Source: CAD feature listing. Evaluate the final solid. Frame: model axes, mm. A direction names the side the tool comes from. Round coordinates to 2 decimals unless told otherwise and drop trailing zeros. Write each loop counter-clockwise with the first axis right and the second up, starting at its lowest first coordinate (ties: lowest second). Pieces come first, ordered by that corner, then holes. Notation, with made-up numbers: M -21.5,32.5 L 1.5,32.5 A11 ccw 1.5,39.5 Z; hole C 9,31 d5. An arc over 180 degrees is marked long. Put each result on its own line as item: value. Start each with the question number.
Autodesk Inventor part; units mm, degrees
ref_plane "YZ Plane" through (0, 0, 0) normal (1, 0, 0) x (0, 1, 0)
ref_plane "XZ Plane" through (0, 0, 0) normal (0, 1, 0) x (-1, 0, 0)
ref_plane "XY Plane" through (0, 0, 0) normal (0, 0, 1) x (1, 0, 0)
sketch "Sketch1" plane through (0, 0, 0) normal (0, 1, 0) x (-1, 0, 0)
  circle A0 centre (0, 0) radius 11.1125
  line L0 (0, -228.6) -> (0, 0) construction
  line L1 (15.875, -228.6) -> (0, -228.6) construction
  circle A1 centre (15.875, -228.6) radius 12.7
  line L2 (25.4, -47.8506) -> (25.4, -198.0228)
  line L3 (57.15, -47.8506) -> (57.15, -181.2924)
  arc A2 (11.2253, 11.2253) -> (-11.2253, -11.2253) centre (0, 0) ccw
  line L4 (-11.2253, -11.2253) -> (25.4, -47.8506)
  arc A3 (57.15, -47.8506) -> (47.8506, -25.4) centre (25.4, -47.8506) ccw
  line L5 (47.8506, -25.4) -> (11.2253, 11.2253)
  circle A4 centre (64.5922, -200.2282) radius 2.8067
  circle A5 centre (64.5922, -256.9718) radius 2.8067
  line L6 (64.5922, -256.9718) -> (64.5922, -200.2282) construction
  line L7 (15.875, -228.6) -> (64.5922, -228.6) construction
  line L8 (15.875, -228.6) -> (-32.8422, -228.6) construction
  circle A6 centre (-32.8422, -228.6) radius 2.8067
  arc A7 (-34.6377, -219.2458) -> (-34.6377, -237.9542) centre (-32.8422, -228.6) ccw
  arc A8 (59.4685, -265.0013) -> (72.1876, -251.2241) centre (64.5922, -256.9718) ccw
  arc A9 (72.1876, -205.9759) -> (65.6336, -190.7603) centre (64.5922, -200.2282) ccw
  line L9 (15.875, -247.65) -> (-34.6377, -237.9542)
  line L10 (15.875, -247.65) -> (15.875, -228.6) construction
  arc A10 (59.4685, -265.0013) -> (15.875, -247.65) centre (-7.6434, -370.1755) ccw
  arc A11 (72.1876, -205.9759) -> (72.1876, -251.2241) centre (102.0848, -228.6) ccw
  arc A12 (57.15, -181.2924) -> (65.6336, -190.7603) centre (66.675, -181.2924) ccw
  line L11 (-34.6377, -219.2458) -> (15.875, -209.55)
  arc A13 (15.875, -209.55) -> (25.4, -198.0228) centre (13.6624, -198.0228) ccw
  line L12 (15.875, -228.6) -> (15.875, -209.55) construction
  line L13 (15.875, -228.6) -> (0, 0) construction
  line L14 (5.5429, -79.8178) -> (46.7187, -76.9583) construction
  circle A14 centre (46.7187, -76.9583) radius 1.905
  line L15 (74.1172, -266.4968) -> (-42.3672, -266.4968) construction
  line L16 (-42.3672, -266.4968) -> (-42.3672, 15.875) construction
  line L17 (-42.3672, 15.875) -> (74.1172, 15.875) construction
  line L18 (74.1172, 15.875) -> (74.1172, -266.4968) construction
  dimension "d0" = 22.225
  dimension "d2" = 228.6
  dimension "d7" = 25.4
  dimension "d17" = 31.75
  dimension "d18" = 45
  dimension "d20" = 25.4
  dimension "d21" = 56.7436
  dimension "d22" = 5.6134
  dimension "d23" = 48.7172
  dimension "d24" = 48.7172
  dimension "d25" = 9.525
  dimension "d26" = 19.05
  dimension "d27" = 19.05
  dimension "d28" = 15.875
  dimension "d29" = 3.81
  dimension "d31" = 41.275
  dimension "d32" = 80.01
  dimension "d33" = 282.3718
  dimension "d34" = 116.4844
extrude "Extrusion1" add sketch "Sketch1" along normal blind 6.35
equation "\"d24\" = d23"
equation "\"d27\" = d26"
properties part number "Intake Arms"
(1) Contact query for flat-ended pins moving along their axis: P1, Ø1.5, axis at y = 3, z = -206, coming from the +X side; P2, Ø7.5, axis at x = -64.59, z = -200.23, coming from the -Y side; P3, Ø2, axis at x = 11.5, y = 2, coming from the -Z side; P4, Ø3, axis at y = 4.5, z = -105, coming from the +X side. Output: stop coordinate, or through.
(2) Section query A-A (z = -228.6). Count the separate pieces of the cut face and the enclosed holes in it, and give its area (3 significant figures).
(3) Ray query, line 1 along Z through (x, y) = (-8.5, 3); line 2 along X through (y, z) = (3.5, -226.5); line 3 along X through (y, z) = (1.5, -108). Return the intervals inside material, ascending.
(4) Section query B-B (x = 1). Return loops of the section in (y, z).
(5) Access query for faces 1 (the flat face through (9.735, 3.131, -214.466)), 2 (the flat face through (-37, 0, -135)). Directions: +Z, -Z, +X, -X, +Y, -Y. A direction counts if a zero-diameter tool reaches every point of the face in a straight line with its end or side. Return the directions, or none.
(6) Pull-direction query (Z, two-part tool) for faces 3 (the cylindrical face through (-22.783, 3.131, -205.412)), 4 (the flat face through (-57.15, 3, -114)), 5 (the flat face through (-29.79, 3.13, -7.34)); classes: +Z half, -Z half, draft (parallel to the pull), parting line (faces both ways), or undercut.
(7) Section query C-C (z = 0). Return loops of the section in (x, y).
Entries:
1. P1: x = -21.51
1. P2: y = 0
1. P3: z = -242.59
1. P4: x = -25.4
2. separate pieces: 3
2. enclosed holes: 0
2. area: 482 mm2
3. line 1: -246.23 to -238.94, -218.26 to -210.97, -30.95 to -7.16, 7.16 to 13.41
3. line 2: -64.65 to -28.4, -3.35 to 30.98, 34.7 to 42.13
3. line 3: -57.15 to -25.4
4. outline: M 0,-244.41 L 6.35,-244.41 L 6.35,-212.79 L 0,-212.79 Z; M 0,-21.45 L 6.35,-21.45 L 6.35,-11.07 L 0,-11.07 Z; M 0,11.07 L 6.35,11.07 L 6.35,15.84 L 0,15.84 Z
5. face 1: +X, +Y, -Y
5. face 2: +Z, -Z, +X, -X, -Y
6. face 3: undercut
6. face 4: draft
6. face 5: +Z half
7. outline: M -22.45,0 L -11.11,0 L -11.11,6.35 L -22.45,6.35 Z; M 11.11,0 L 15.87,0 L 15.87,6.35 L 11.11,6.35 Z
